The drawing under review shows one solid part. Ordinate dimensions are in mm from its lowest x, y, z. A direction names the side the tool comes from. Round coordinates to 2 decimals unless told otherwise and drop trailing zeros. Order: outer loops, then holes, each group sorted by start corner. A loop starts at its lowest first (then second) coordinate and runs counter-clockwise, first axis right, second up. Notation, with made-up numbers: (46.25, 40) - (82.25, 40) arc R29 cw to (82.25, 63) - close; hole circle Ø8 at (5, 38.25). An arc over 180 degrees is marked (long way). One line per question, with ' | ' between items.
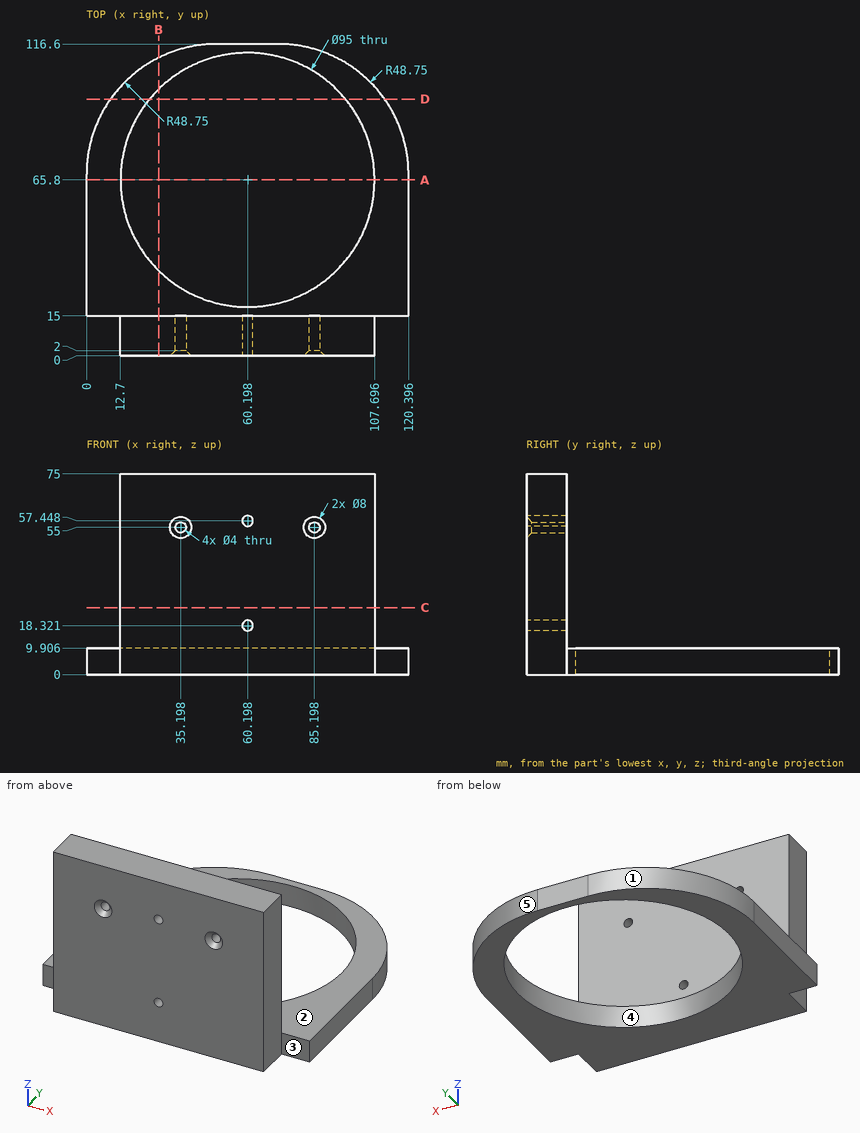
(1) We need section B-B on x = 27. State the section outline as (y, z) points (1 decimal), plus the area to 3 significant figures.
Output values:
outline: (0, 0) - (31.8, 0) - (31.8, 9.9) - (15, 9.9) - (15, 75) - (0, 75) - close; (99.8, 0) - (111.5, 0) - (111.5, 9.9) - (99.8, 9.9) - close | area: 1,410 mm^2
(2) We need section C-C on z = 25. State the section outline as (x, y) points (1 decimal), plus the area to 4 significant figures.
Output values:
outline: (12.7, 0) - (107.7, 0) - (107.7, 15) - (12.7, 15) - close | area: 1,425 mm^2
(3) We need section D-D on y = 96. State the section outline as (x, z) points (1 decimal), plus the area to 3 significant figures.
Output values:
outline: (8.9, 0) - (23.5, 0) - (23.5, 9.9) - (8.9, 9.9) - close; (96.9, 0) - (111.4, 0) - (111.4, 9.9) - (96.9, 9.9) - close | area: 289 mm^2
(4) For probe 1 along X at (y, z) = (8.75, 55) (1 decimal); probe 2 along Z at (x, y) = (111, 27) (1 decimal); probe 3 along Y at (x, z) = (70.5, 66.5), list the stretches that pass through material, from the lowest coordinate up. Write a range as [from, to].
Output values:
probe 1: [12.7, 33.2], [37.2, 83.2], [87.2, 107.7] | probe 2: [0, 9.9] | probe 3: [0, 15]
(5) For the marked faces 1 and 2, list the 3-axis set-ups (+Z, -Z, +X, -X, +Y, -Y) from which the entire face can be reached by the end or side of a thin tool; tool diameter is ignored.
Output values:
face 1: +Z, -Z, -X, +Y | face 2: +Z, +X, -X, +Y
(6) Insertion check: pin 1 (4.5 mm diameter, centred on x = 35.198, z = 55, fed in from +Y); pin 2 (8 mm diameter, centred on x = 7.5, z = 4, fed in from -Y); pin 3 (7.5 mm diameter, centred on y = 10.5, z = 37, fed in from +X). Each pin has a flat end and moves straight along its axis. Give the tip position at first contact, or say it passes through.
Output values:
pin 1: y = 15 | pin 2: y = 15 | pin 3: x = 107.7
(7) We need section A-A on y = 65.8. State the section outline as (x, z) points (1 decimal).
Output values:
outline: (0, 0) - (12.7, 0) - (12.7, 9.9) - (0, 9.9) - close; (107.7, 0) - (120.4, 0) - (120.4, 9.9) - (107.7, 9.9) - close
(8) Mouldability with a two-part tool opening along X and no side actions: class the marked faces 3, 4 and 5 as released by +X, released by -X, zero draft, split by the parting line, or undercut.
Output values:
face 3: zero draft | face 4: undercut | face 5: released by +X
